Solid Edge part; units mm, degrees
sketch "Sketch1" plane through (0, 0, 0) normal (0, 0, 1) x (1, 0, 0)
  line L0 (-47.5, 5) -> (-47.5, -5)
  line L1 (-47.5, -5) -> (47.5, -5)
  line L2 (47.5, -5) -> (47.5, 5)
  line L3 (47.5, 5) -> (-47.5, 5)
  dimension "D1" = 47.5
  dimension "D2" = 47.5
extrude "Ajout_matière_1" add sketch "Sketch1" along normal blind 2.25
sketch "Sketch2" plane through (0, 0, 2.25) normal (0, 0, 1) x (1, 0, 0)
  line L0 (-47.5, 5) -> (-47.5, -5)
  line L1 (-47.5, -5) -> (-37.5, -5)
  line L2 (-37.5, -5) -> (-37.5, 5)
  line L3 (-37.5, 5) -> (-47.5, 5)
  dimension "D1" = 37.5
extrude "Ajout_matière_2" add sketch "Sketch2" along normal blind 8
sketch "Sketch3" plane through (-42.5, 0, 10.25) normal (0, 0, 1) x (1, 0, 0)
  circle A0 centre (0, 0) radius 1.5
extrude "Enlèvement_matière_1" cut sketch "Sketch3" against normal blind 5
sketch "Sketch4" plane through (0, -5, 6) normal (0, -1, 0) x (1, 0, 0)
  circle A0 centre (-42.5, 0.25) radius 2
extrude "Enlèvement_matière_2" cut sketch "Sketch4" against normal blind 10
sketch "Sketch5" plane through (7.5, 0, 2.25) normal (0, 0, 1) x (1, 0, 0)
  line L0 (-13.5, 5) -> (-1.5, 5)
  line L1 (-1.5, 5) -> (-1.5, -5)
  line L2 (-1.5, -5) -> (-13.5, -5)
  line L3 (-13.5, -5) -> (-13.5, 5)
  dimension "D1" = 13.5
extrude "Ajout_matière_3" add sketch "Sketch5" along normal blind 8
sketch "Sketch6" plane through (0, 0, 10.25) normal (0, 0, 1) x (1, 0, 0)
  circle A0 centre (0, 0) radius 2.5
extrude "Enlèvement_matière_3" cut sketch "Sketch6" against normal blind 11
fillet "Congé_2" radius 1 2 edges at (-47.5, 0, 0) (-47.5, 0, 10.25)
sketch "Sketch7" plane through (33.649, 0, 2.25) normal (0, 0, 1) x (1, 0, 0)
  line L0 (13.851, 5) -> (13.851, -5)
  arc A0 (13.851, 5) -> (13.851, -5) centre (13.851, 0) cw
extrude "Ajout_matière_4" add sketch "Sketch7" against normal blind 2.25
fillet "Congé_3" radius 10 3 edges at (-37.5, 0, 2.25) (-6, 0, 2.25) (6, 0, 2.25)
properties material "Plastique ABS, haute performance"
For this review, take the finished solid that the model builds, in its own axes (mm). A direction names the side the tool comes from. Round coordinates to 2 decimals unless told otherwise and drop trailing zeros. Loops run counter-clockwise (first coordinate to the right, second up) from the corner with the lowest first, then second, coordinate; pieces in that order, holes last. Notation, with made-up numbers: (39, 59) - (75, 59) arc R19 cw to (75, 75) - close; hole circle Ø10 at (66, 53.25). An arc over 180 degrees is marked (long way). Use one line per item in the form item = value.
1) We need section A-A on y = 0. Write out the cut boundary in (x, z).
Solutions:
outline = (-47.5, 1) arc R1 ccw to (-46.5, 0) - (-2.5, 0) - (-2.5, 10.25) - (-6, 10.25) arc R10 cw to (-15.8, 2.25) - (-27.7, 2.25) arc R10 cw to (-37.5, 10.25) - (-41, 10.25) - (-41, 7.57) arc R2 cw (long way) to (-44, 7.57) - (-44, 10.25) - (-46.5, 10.25) arc R1 ccw to (-47.5, 9.25) - close; (2.5, 0) - (52.5, 0) - (52.5, 2.25) - (15.8, 2.25) arc R10 cw to (6, 10.25) - (2.5, 10.25) - close
2) Clearance check with flat-ended pins moving along their axes: P1, Ø5, axis at x = -32.5, y = -2.5, coming from the -Z side; P2, Ø3, axis at x = 43, y = -1.5, coming from the +Z side; P3, Ø6, axis at y = -1.5, z = 9, coming from the +X side. State where each tip first meets the part, or that it passes through.
Solutions:
P1 = 0
P2 = 2.25
P3 = 7.99
3) We need section C-C on z = 6.25. Write out the cut boundary in (x, y), then the cut area to 3 significant figures.
Solutions:
outline = (-47.5, -5) - (-44.5, -5) - (-44.5, 5) - (-47.5, 5) - close; (-40.5, -5) - (-35.7, -5) - (-35.7, 5) - (-40.5, 5) - close; (-7.8, -5) - (7.8, -5) - (7.8, 5) - (-7.8, 5) - close; hole circle Ø5 at (0, 0)
area = 214 mm2
4) Mouldability with a two-part tool opening along Y and no side actions: class faces 1 (the face through (-22, 0, 2.25)), 2 (the face through (-41, 0, 9)), 3 (the face through (-10, 5, 3)) as pulls with the +Y half, pulls with the -Y half, needs draft (parallel to the pull), parting line crosses it, or undercut.
Solutions:
face_1 = needs draft
face_2 = undercut
face_3 = pulls with the +Y half
5) We need section B-B on x = 0. Write out the cut boundary in (y, z).
Solutions:
outline = (-5, 0) - (-2.5, 0) - (-2.5, 10.25) - (-5, 10.25) - close; (2.5, 0) - (5, 0) - (5, 10.25) - (2.5, 10.25) - close
6) We need section D-D on y = -4. Write out the cut boundary in (x, z), then the cut area to 3 significant figures.
Solutions:
outline = (-47.5, 1) arc R1 ccw to (-46.5, 0) - (50.5, 0) - (50.5, 2.25) - (15.8, 2.25) arc R10 cw to (6, 10.25) - (-6, 10.25) arc R10 cw to (-15.8, 2.25) - (-27.7, 2.25) arc R10 cw to (-37.5, 10.25) - (-46.5, 10.25) arc R1 ccw to (-47.5, 9.25) - close; hole circle Ø4 at (-42.5, 6.25)
area = 443 mm2
7) Tool access review of faces 4 (the face through (-34.101, -0.07, 4.565)), 5 (the face through (34, 0, 2.25)), 6 (the face through (-0.54, -2.44, 5.2)): name each direction out of +Z, -Z, +X, -X, +Y, -Y from which nothing blocks a thin tool from reaching the whole face with its end or side.
Solutions:
face_4 = +Z, +Y, -Y
face_5 = +Z, +X, +Y, -Y
face_6 = +Z, -Z
8) Wall thickness on probe 1 along Y at (x, z) = (0, 7.5); probe 2 along Z at (x, y) = (-42.5, 3.25); probe 3 along X at (y, z) = (-3.25, 7.5): over which ranges is each line inside the solid? List them lowest first.
Solutions:
probe_1 = -5 to -2.5, 2.5 to 5
probe_2 = 0 to 4.25, 8.25 to 10.25
probe_3 = -47.5 to -44.06, -40.94 to -36.5, -7 to 7
